For this review, take the finished solid that the model builds, in its own axes (mm). A direction names the side the tool comes from. Round coordinates to 2 decimals unless told otherwise and drop trailing zeros. Write each loop counter-clockwise with the first axis right and the second up, starting at its lowest first coordinate (ties: lowest second). Pieces come first, ordered by that corner, then holes. Notation, with made-up numbers: (60.5, -34.5) -> (99.5, -34.5) arc R7 ccw to (99.5, -26.5) -> close; hole circle Ø7 at (-15.75, 66.5). An arc over 180 degrees is marked (long way). Answer in a Markdown table with one row per item. Add a question column.
Autodesk Fusion 360 part; units mm, degrees
sketch "Sketch1" plane through (0, 0, 0) normal (0, 0, 1) x (1, 0, 0)
  circle A0 centre (0, 0) radius 6
  dimension "d1" = 12
ref_plane "WorkPlane1" through (0, 0, -9) normal (0, 0, 1) x (1, 0, 0)
sketch "Sketch3" plane through (0, 0, -9) normal (0, 0, 1) x (1, 0, 0)
  circle A0 centre (0, 0) radius 6.5
  dimension "d8" = 13
sketch "Sketch4" plane through (0, 0, -9) normal (0, 0, 1) x (1, 0, 0)
  circle A0 centre (0, 0) radius 5
  dimension "d9" = 10
loft "Loft1" add profiles "Sketch3", "Sketch1" section 1 section 2
extrude "Extrude3" add sketch "Sketch4" against normal blind 160
sketch "Sketch5" plane through (0, 0, -169) normal (0, 0, -1) x (1, 0, 0)
  circle A0 centre (0, 0) radius 5
  circle A1 centre (0, 0) radius 4.5
  dimension "d12" = 9
extrude "Extrude4" add sketch "Sketch5" along normal blind 36 contours A1
1. We need section A-A (x = 0). Write out the cut boundary in (y, z), plus the area to 3 significant figures.
2. Clearance check with flat-ended pins moving along their axes: pin 1 Ø6 at (x, z) = (3, -112) entering from -Y; pin 2 Ø1.5 at (y, z) = (4.5, -92.5) entering from +X; pin 3 Ø1.5 at (y, z) = (5, -41) entering from -X. State where each tip first meets the part, or that it passes through.
3. For L1, parallel to Z at x = -4.25, y = -2.75; L2, parallel to Y at x = -2.25, z = -121; L3, parallel to Y at x = 0, z = -68, list the stretches that pass through material, from the lowest coordinate up. Write a range as [from, to].
4. We need section B-B (z = -99). Write out the cut boundary in (x, y), plus the area to 3 significant figures.
5. Tool access review of faces 1 (the cylindrical face through (-0.59, 4.46, -186.75)), 2 (the conical face through (-4.96, 3.81, -4.56)): name each direction out of +Z, -Z, +X, -X, +Y, -Y from which nothing blocks a thin tool from reaching the whole face with its end or side.
Response:
| question | item | result |
|---|---|---|
| 1 | outline | (-6.5, -9) -> (-5, -9) -> (-5, -169) -> (-4.5, -169) -> (-4.5, -205) -> (4.5, -205) -> (4.5, -169) -> (5, -169) -> (5, -9) -> (6.5, -9) -> (6, 0) -> (-6, 0) -> close |
| 1 | area | 2,040 mm2 |
| 2 | pin 1 | y = -5 |
| 2 | pin 2 | x = 3.31 |
| 2 | pin 3 | x = -2.63 |
| 3 | L1 | [-9, 0] |
| 3 | L2 | [-4.47, 4.47] |
| 3 | L3 | [-5, 5] |
| 4 | outline | circle Ø10 at (0, 0) |
| 4 | area | 78.5 mm2 |
| 5 | face 1 | -Z |
| 5 | face 2 | +Z |
